Job drawing, mm, ordinate dimensions from the low corner. One solid piece. A direction names the side the tool comes from. Round coordinates to 2 decimals unless told otherwise and drop trailing zeros. Loops run counter-clockwise (first coordinate to the right, second up) from the corner with the lowest first, then second, coordinate; pieces in that order, holes last. Notation, with made-up numbers: M 62.25,51 L 101.25,51 A26 cw 101.25,83 Z; hole C 80,76 d5. An arc over 180 degrees is marked long. One line per item, written item: value.
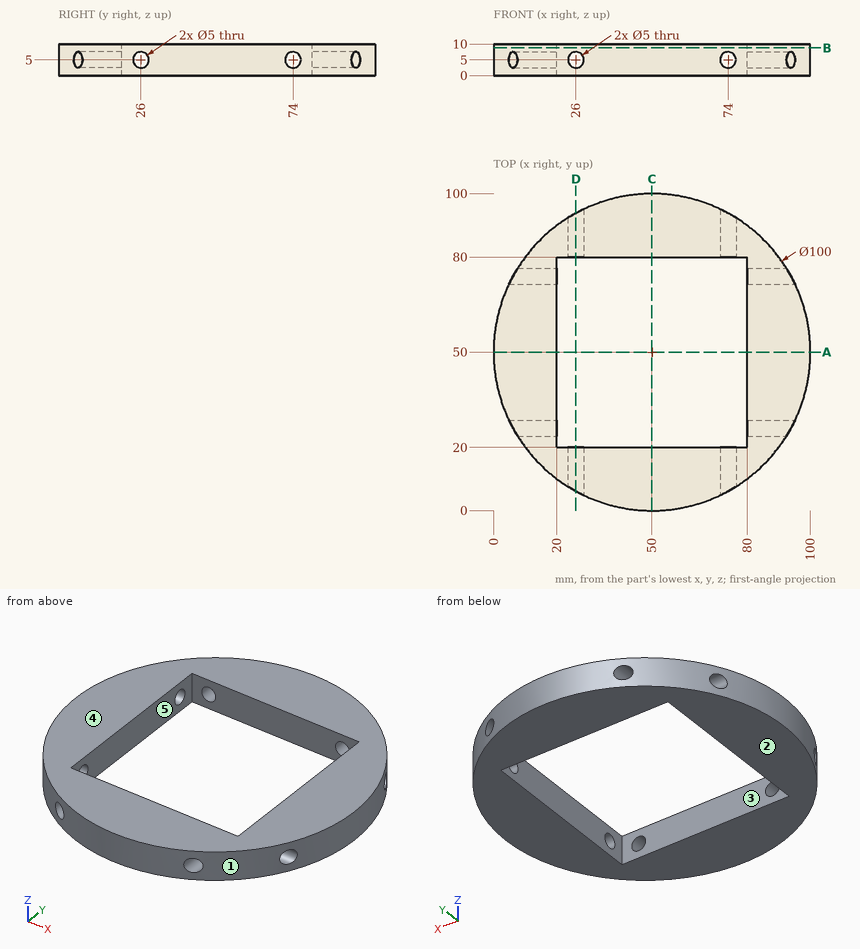
Item 1: Slice it at D-D, the plane x = 26. Give the cut face in (y, z).
Check values:
outline: M 6.14,0 L 20,0 L 20,2.5 L 6.14,2.5 Z; M 6.14,7.5 L 20,7.5 L 20,10 L 6.14,10 Z; M 80,0 L 93.86,0 L 93.86,2.5 L 80,2.5 Z; M 80,7.5 L 93.86,7.5 L 93.86,10 L 80,10 Z
Item 2: Slice it at B-B, the plane z = 8.75. Give the cut face in (x, y).
Check values:
outline: C 50,50 d100; hole M 20,20 L 80,20 L 80,80 L 20,80 Z
Item 3: Wall check: line 1 along Z through (x, y) = (16, 74); line 2 along X through (y, z) = (49.5, 5.75); line 3 along Y through (x, z) = (82.5, 4.75). Give the ranges that are in metal, low to high.
Check values:
line 1: z = 0 to 2.5, 7.5 to 10
line 2: x = 0 to 20, 80 to 100
line 3: y = 12 to 23.51, 28.49 to 71.51, 76.49 to 88
Item 4: Drop flat-ended pins along their axis: P1, Ø1.5, axis at x = 13.5, z = 4.5, coming from the -Y side; P2, Ø3, axis at x = 46, z = 3.5, coming from the +Y side; P3, Ø6, axis at x = 74, z = 5, coming from the -Y side. Give the stop position or say it passes through.
Check values:
P1: stops at y = 15.04
P2: stops at y = 99.94
P3: stops at y = 4.62
Item 5: Slice it at A-A, the plane y = 50. Give the cut face in (x, z).
Check values:
outline: M 0,0 L 20,0 L 20,10 L 0,10 Z; M 80,0 L 100,0 L 100,10 L 80,10 Z
Item 6: Pull direction X, two halves, no side cores. Call the marked faces 1, 2 and 3: pulls with the +X half, pulls with the -X half, needs draft (parallel to the pull), parting line crosses it, or undercut.
Check values:
face 1: parting line crosses it
face 2: needs draft
face 3: undercut
Item 7: Which spindle directions (+Z, -Z, +X, -X, +Y, -Y) get a long thin tool onto all of the face, cutting with end or side? Do the marked faces 4 and 5. Say none if no direction does.
Check values:
face 4: +Z, +X, -X, +Y, -Y
face 5: +Z, -Z
